Job drawing, mm, ordinate dimensions from the low corner. One solid piece. A direction names the side the tool comes from. Give positions to 0.01 mm unless a question says otherwise; leave off trailing zeros. Loops run counter-clockwise (first coordinate to the right, second up) from the corner with the lowest first, then second, coordinate; pieces in that order, holes last.
Item 1: Drop flat-ended pins along their axis: P1, Ø5, axis at x = 9.5, z = 4.5, coming from the +Y side; P2, Ø3, axis at y = 4.5, z = 10.5, coming from the -X side; P3, Ø4, axis at x = 10, z = 7.5, coming from the +Y side; P4, Ø1, axis at y = 3, z = 5, coming from the +X side. Give the stop position or say it passes through.
Item 2: Which spindle directions (+Z, -Z, +X, -X, +Y, -Y) get a long thin tool onto all of the face, cutting with end or side? Do the marked faces 1 and 2. Say none if no direction does.
Item 3: Saw through at C-C on x = 3.5. Give the cut face in (y, z).
Item 4: Mould opens along X. For the marked faces 3, 4, 5 and 6 say: released by +X, released by -X, zero draft, split by the parting line, or undercut.
Item 5: Saw through at A-A on z = 6. Give the cut face in (x, y).
Item 6: Probe probe 1 along Z at (x, y) = (10, 5.65); probe 2 along Y at (x, z) = (9.5, 6.75); probe 3 along Y at (x, z) = (2.25, 3.25). List the from-to ranges inside material, lowest first.
Item 7: Saw through at D-D on z = 4.5. Give the cut face in (x, y), plus the area to 3 significant figures.
Item 8: Saw through at B-B on y = 3.5. Give the cut face in (x, z).
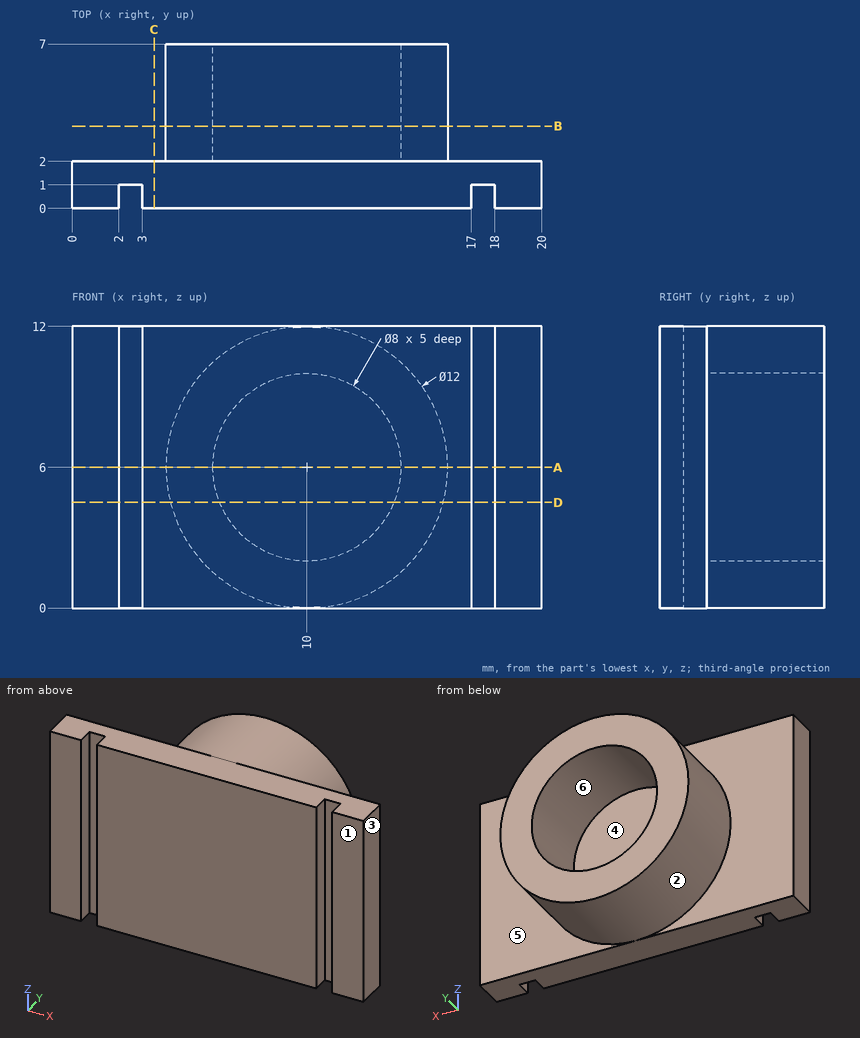
Results below:
1. P1: stops at y = 7
1. P2: stops at x = 4.8
1. P3: stops at y = 2
1. P4: stops at x = 15.98
2. face 1: +Z, -Z, +X, -X, -Y
2. face 2: +Y
3. outline: (0, 0) - (2, 0) - (2, 12) - (0, 12) - close
4. face 3: released by +X
4. face 4: undercut
4. face 5: zero draft
4. face 6: undercut
5. outline: (0, 0) - (2, 0) - (2, 1) - (3, 1) - (3, 0) - (17, 0) - (17, 1) - (18, 1) - (18, 0) - (20, 0) - (20, 2) - (16, 2) - (16, 7) - (14, 7) - (14, 2) - (6, 2) - (6, 7) - (4, 7) - (4, 2) - (0, 2) - close
6. probe 1: z = 0 to 2, 10 to 12
6. probe 2: y = 0 to 2
6. probe 3: y = 1 to 2
7. outline: (0, 0) - (2, 0) - (2, 1) - (3, 1) - (3, 0) - (17, 0) - (17, 1) - (18, 1) - (18, 0) - (20, 0) - (20, 2) - (15.81, 2) - (15.81, 7) - (13.71, 7) - (13.71, 2) - (6.29, 2) - (6.29, 7) - (4.19, 7) - (4.19, 2) - (0, 2) - close
7. area: 59.0 mm2
8. outline: circle Ø12 at (10, 6); hole circle Ø8 at (10, 6)
